from build123d import *

# Parameters (mm, degrees)
AUFSATZ_LINEAR_AUSTRAGEN1_DEPTH = 10


with BuildPart() as part:
    # Skizze2 → Aufsatz-Linear austragen1 (new body)
    with BuildSketch(Plane(origin=(0, 0, 0), x_dir=(1, 0, 0), z_dir=(0, 1, 0))):
        with BuildLine():
            Line((0, 0), (0, 55.62))
            ThreePointArc((0, 55.62), (0.439339828, 56.680660172), (1.5, 57.12))
            Line((1.5, 57.12), (17.54, 57.12))
            ThreePointArc((17.54, 57.12), (18.600660172, 57.559339828), (19.04, 58.62))
            Line((19.04, 58.62), (19.04, 62.76))
            ThreePointArc((19.04, 62.76), (19.479339828, 63.820660172), (20.54, 64.26))
            Line((20.54, 64.26), (104.098679656, 64.26))
            ThreePointArc((104.098679656, 64.26), (104.672704805, 64.145819299), (105.159339828, 63.820660172))
            Line((105.159339828, 63.820660172), (109.040660172, 59.939339828))
            ThreePointArc((109.040660172, 59.939339828), (109.527295195, 59.614180701), (110.101320344, 59.5))
            Line((110.101320344, 59.5), (112.74, 59.5))
            ThreePointArc((112.74, 59.5), (113.800660172, 59.060660172), (114.24, 58))
            Line((114.24, 58), (114.24, 6.708065653))
            ThreePointArc((114.24, 6.708065653), (114.280993169, 6.359785497), (114.401732089, 6.030541484))
            Line((114.401732089, 6.030541484), (123.948031101, -12.825620738))
            ThreePointArc((123.948031101, -12.825620738), (124.109197107, -13.544350864), (123.908801296, -14.253144906))
            Line((123.908801296, -14.253144906), (114.755057795, -30.10789373))
            ThreePointArc((114.755057795, -30.10789373), (114.102280417, -30.71153588), (113.222449486, -30.839597128))
            Line((113.222449486, -30.839597128), (53.266068474, -21.388296602))
            ThreePointArc((53.266068474, -21.388296602), (53.149641138, -21.374581146), (53.032498271, -21.37))
            Line((53.032498271, -21.37), (1.5, -21.37))
            ThreePointArc((1.5, -21.37), (0.439339828, -20.930660172), (0, -19.87))
            Line((0, -19.87), (0, 0))
        make_face()
    extrude(amount=AUFSATZ_LINEAR_AUSTRAGEN1_DEPTH)


solid = part.part
Model file for the job. Use its own axes, mm. A direction names the side the tool comes from. Give positions to 0.01 mm unless a question says otherwise; leave off trailing zeros. Order: outer loops, then holes, each group sorted by start corner. A loop starts at its lowest first (then second) coordinate and runs counter-clockwise, first axis right, second up. Notation, with made-up numbers: M -38,35.25 L -30,35.25 A12 ccw -30,40.25 Z; hole C 44,56.25 d9. An arc over 180 degrees is marked long. Put each result on its own line as item: value. Start each with the question number.
(1) Band-saw the part on B-B on z = -11. Give the cut face in (x, y), then the cut area to 3 significant figures.
(2) Tool access for faces 1 (the face through (9, 5, -57.12)), 2 (the face through (28, 5, 21.37)), 3 (the face through (63, 10, -17)), 4 (the face through (111, 5, -59.5)): list every direction of +Z, -Z, +X, -X, +Y, -Y with a clear straight run to the whole face (end or side of a thin tool).
(3) Band-saw the part on A-A on y = 5.25. Give the cut face in (x, z), then the cut area to 3 significant figures.
(4) Pin check, flat tips, straight feed: pin 1 Ø1 at (y, z) = (8.5, -48.5) entering from +X; pin 2 Ø1.3 at (x, y) = (111.5, 5.5) entering from -Z; pin 3 Ø1.5 at (x, y) = (19, 5) entering from -Z. Stop position of each tip, or through.
(5) Drill centre lines: L1, parallel to Z at x = 21, y = 2; L2, parallel to X at y = 9.75, z = -28.5; L3, parallel to Z at x = 7.5, y = 7.5. Where is each one in solid material? Low to high. Write a range as [from, to].
(6) Band-saw the part on C-C on x = 25. Give the cut face in (y, z), then the cut area to 3 significant figures.
Results below:
1. outline: M 0,0 L 114.24,0 L 114.24,10 L 0,10 Z
1. area: 1,140 mm2
2. face 1: -Z, -X, +Y, -Y
2. face 2: +Z, -X, +Y, -Y
2. face 3: +Z, -Z, +X, -X, +Y
2. face 4: -Z, +X, +Y, -Y
3. outline: M 0,-55.62 A1.5 ccw 1.5,-57.12 L 17.54,-57.12 A1.5 cw 19.04,-58.62 L 19.04,-62.76 A1.5 ccw 20.54,-64.26 L 104.1,-64.26 A1.5 ccw 105.16,-63.82 L 109.04,-59.94 A1.5 cw 110.1,-59.5 L 112.74,-59.5 A1.5 ccw 114.24,-58 L 114.24,-6.71 A1.5 cw 114.4,-6.03 L 123.95,12.83 A1.5 ccw 123.91,14.25 L 114.76,30.11 A1.5 ccw 113.22,30.84 L 53.27,21.39 A1.5 cw 53.03,21.37 L 1.5,21.37 A1.5 ccw 0,19.87 Z
3. area: 10,100 mm2
4. pin 1: stops at x = 114.24
4. pin 2: stops at z = -59.5
4. pin 3: stops at z = -64.04
5. L1: z = [-64.26, 21.37]
5. L2: x = [0, 114.24]
5. L3: z = [-57.12, 21.37]
6. outline: M 0,-64.26 L 10,-64.26 L 10,21.37 L 0,21.37 Z
6. area: 856 mm2
